Input: part model. Units: mm. Frame: model coordinates. Face numbers are marked on the shaded views. A direction names the side the tool comes from. Give positions to 0.01 mm unless a question says otherwise; leave off trailing zeros. Write each loop counter-clockwise with the first axis right and the second up, starting at its lowest first coordinate (ties: lowest second). Pieces come first, ordered by that corner, then holes. Notation, with made-up numbers: (3, 55.5) - (55, 55.5) arc R15 ccw to (55, 81.5) - close; hole circle Ø6 at (-15, 66.25). An arc over 180 degrees is marked (long way). Answer as CSV lines item,"result".
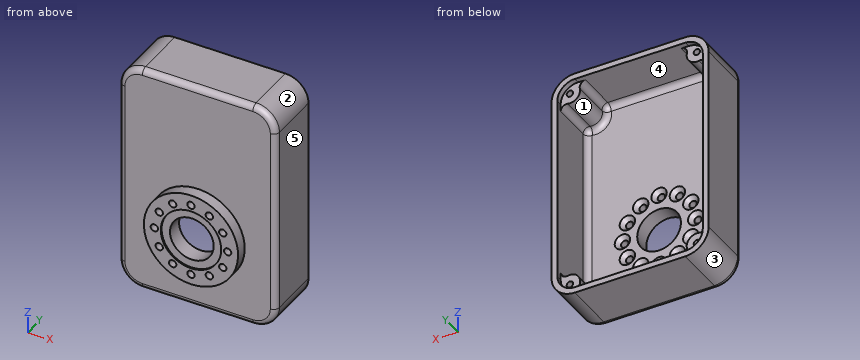
```python
from build123d import *

# Parameters (mm, degrees)
BOSS_EXTRUDE1_START           = 2.54
SKETCH4_R                     = 9.5504
BOSS_EXTRUDE1_DEPTH           = 2.54
CSK_FOR_M3_SFHCS1_D           = 3.2
CSK_FOR_M3_SFHCS1_CSINK_D     = 6.72
CSK_FOR_M3_SFHCS1_CSINK_ANGLE = 90
BOSS_EXTRUDE4_START           = 22.225
BOSS_EXTRUDE4_DEPTH           = 22.225
FILLET1_R                     = 2.54
SKETCH8_R                     = 4.445
SKETCH8_R_2                   = 1.3890625
BOSS_EXTRUDE5_DEPTH           = 19.685
FILLET3_R                     = 2.54
FILLET4_R                     = 2.54


with BuildPart() as part:
    # Sketch1 → Revolve1 (revolve)
    with BuildSketch(Plane.XY, mode=Mode.PRIVATE) as revolve1_sk:
        Polygon((-9.5504, 0), (-20.574, 0), (-20.574, -5.08), (-13.208, -5.08), (-13.208, -4.445), (-9.5504, -4.445), align=None)
    revolve(revolve1_sk.sketch.rotate(Axis((0, 0, 0), (0, 1, 0)), 270), axis=Axis((0, 0, 0), (0, 1, 0)))

    # Sketch4 → Boss-Extrude1 (add)
    with BuildSketch(Plane(origin=(0, 0, 0), x_dir=(1, 0, 0), z_dir=(0, 1, 0)).offset(BOSS_EXTRUDE1_START)):
        with BuildLine():
            Line((-24.13, -67.31), (24.13, -67.31))
            ThreePointArc((24.13, -67.31), (31.314204897, -64.334204897), (34.29, -57.15))
            Line((34.29, -57.15), (34.29, 24.13))
            ThreePointArc((34.29, 24.13), (31.314204897, 31.314204897), (24.13, 34.29))
            Line((24.13, 34.29), (-24.13, 34.29))
            ThreePointArc((-24.13, 34.29), (-31.314204897, 31.314204897), (-34.29, 24.13))
            Line((-34.29, 24.13), (-34.29, -57.15))
            ThreePointArc((-34.29, -57.15), (-31.314204897, -64.334204897), (-24.13, -67.31))
        make_face()
        Circle(SKETCH4_R, mode=Mode.SUBTRACT)
    extrude(amount=-BOSS_EXTRUDE1_DEPTH)

    # CSK for M3 SFHCS1 (through all)
    with Locations(Plane(origin=(0, 2.54, 0), x_dir=(1, 0, 0), z_dir=(0, 1, 0))):
        with Locations((-13.858138511, -8.001), (-16.002, 0), (-13.858138511, 8.001), (-8.001, 13.858138511), (0, 16.002), (8.001, 13.858138511), (13.858138511, 8.001), (16.002, 0), (13.858138511, -8.001), (8.001, -13.858138511), (0, -16.002), (-8.001, -13.858138511)):
            CounterSinkHole(CSK_FOR_M3_SFHCS1_D / 2, CSK_FOR_M3_SFHCS1_CSINK_D / 2, counter_sink_angle=CSK_FOR_M3_SFHCS1_CSINK_ANGLE)

    # Sketch6 → Boss-Extrude4 (add)
    with BuildSketch(Plane(origin=(0, 2.54, 0), x_dir=(1, 0, 0), z_dir=(0, 1, 0)).offset(BOSS_EXTRUDE4_START)):
        with BuildLine():
            Line((24.13, 34.29), (-24.13, 34.29))
            ThreePointArc((-24.13, 34.29), (-31.314204897, 31.314204897), (-34.29, 24.13))
            Line((-34.29, 24.13), (-34.29, -57.15))
            ThreePointArc((-34.29, -57.15), (-31.314204897, -64.334204897), (-24.13, -67.31))
            Line((-24.13, -67.31), (24.13, -67.31))
            ThreePointArc((24.13, -67.31), (31.314204897, -64.334204897), (34.29, -57.15))
            Line((34.29, -57.15), (34.29, 24.13))
            ThreePointArc((34.29, 24.13), (31.314204897, 31.314204897), (24.13, 34.29))
        make_face()
        with BuildLine():
            Line((24.13, 31.75), (-24.13, 31.75))
            ThreePointArc((-24.13, 31.75), (-29.518153673, 29.518153673), (-31.75, 24.13))
            Line((-31.75, 24.13), (-31.75, -57.15))
            ThreePointArc((-31.75, -57.15), (-29.518153673, -62.538153673), (-24.13, -64.77))
            Line((-24.13, -64.77), (24.13, -64.77))
            ThreePointArc((24.13, -64.77), (29.518153673, -62.538153673), (31.75, -57.15))
            Line((31.75, -57.15), (31.75, 24.13))
            ThreePointArc((31.75, 24.13), (29.518153673, 29.518153673), (24.13, 31.75))
        make_face(mode=Mode.SUBTRACT)
    extrude(amount=-BOSS_EXTRUDE4_DEPTH)

    # Fillet1
    fillet1_edges = [part.edges().sort_by_distance(p)[0] for p in [
        (-31.314204897, 0, 64.334204897),
        (0, 0, 67.31),
        (31.314204897, 0, 64.334204897),
        (34.29, 0, 16.51),
        (31.314204897, 0, -31.314204897),
        (0, 0, -34.29),
        (-31.314204897, 0, -31.314204897),
        (-34.29, 0, 16.51),
    ]]
    fillet(fillet1_edges, radius=FILLET1_R)

    # Sketch8 → Boss-Extrude5 (add)
    # profile 1 of 4: a face of its own
    with BuildSketch(Plane(origin=(0, 2.54, 0), x_dir=(1, 0, 0), z_dir=(0, 1, 0))):
        with Locations((-27.722102448, -60.742102448)):
            Circle(SKETCH8_R)
        with Locations(Location((-27.722102448, -60.742102448, 0), (0, 0, 270))):
            Circle(SKETCH8_R_2, mode=Mode.SUBTRACT)
    # profile 2 of 4: a face of its own
    with BuildSketch(Plane(origin=(0, 2.54, 0), x_dir=(1, 0, 0), z_dir=(0, 1, 0))):
        with Locations((27.722102448, -60.742102448)):
            Circle(SKETCH8_R)
        with Locations(Location((27.722102448, -60.742102448, 0), (0, 0, 270))):
            Circle(SKETCH8_R_2, mode=Mode.SUBTRACT)
    # profile 3 of 4: a face of its own
    with BuildSketch(Plane(origin=(0, 2.54, 0), x_dir=(1, 0, 0), z_dir=(0, 1, 0))):
        with Locations((27.722102448, 27.722102448)):
            Circle(SKETCH8_R)
        with Locations(Location((27.722102448, 27.722102448, 0), (0, 0, 270))):
            Circle(SKETCH8_R_2, mode=Mode.SUBTRACT)
    # profile 4 of 4: a face of its own
    with BuildSketch(Plane(origin=(0, 2.54, 0), x_dir=(1, 0, 0), z_dir=(0, 1, 0))):
        with Locations((-27.722102448, 27.722102448)):
            Circle(SKETCH8_R)
        with Locations(Location((-27.722102448, 27.722102448, 0), (0, 0, 270))):
            Circle(SKETCH8_R_2, mode=Mode.SUBTRACT)
    extrude(amount=BOSS_EXTRUDE5_DEPTH)

    # Fillet3
    # the kernel refuses this fillet: 2.54 mm, written as the material it adds along each edge
    with BuildSketch(Plane(origin=(25.571770391, 2.54, 64.632359129), x_dir=(-0.5973974080073474, 0, -0.8019453453360166), z_dir=(0, 1, 0)), Plane(origin=(31.612359129, 2.54, -25.571770391), x_dir=(-0.8019453453360167, 0, 0.5973974080073472), z_dir=(0, 1, 0)), Plane(origin=(-25.571770391, 2.54, -31.612359129), x_dir=(0.5973974080073424, 0, 0.8019453453360202), z_dir=(0, 1, 0)), Plane(origin=(-31.612359129, 2.54, 58.591770391), x_dir=(0.8019453453360194, 0, -0.5973974080073438), z_dir=(0, 1, 0))) as fillet3_piece_1:
        with BuildLine():
            CenterArc((4.719009703, 2.313416024), FILLET3_R, 143.316272758, 102.298995101)
            Line((2.682068526, 3.83080544), (2.478374408, 3.982544382))
            ThreePointArc((2.478374408, 3.982544382), (0.547235321, 1.390186295), (-0.228725099, 0.110457363))
            Line((-0.228725099, 0.110457363), (0.104866882, -0.231341602))
            ThreePointArc((0.104866882, -0.231341602), (1.83517044, 0.142521958), (3.565473998, -0.231341602))
            Line((3.565473998, -0.231341602), (3.67034088, 0))
        make_face()
    extrude(amount=19.685)
    with BuildSketch(Plane(origin=(31.612359129, 2.54, 58.591770391), x_dir=(-0.8019453453360176, 0, -0.5973974080073462), z_dir=(0, 1, 0)), Plane(origin=(25.571770391, 2.54, -31.612359129), x_dir=(-0.5973974080073442, 0, 0.801945345336019), z_dir=(0, 1, 0)), Plane(origin=(-31.612359129, 2.54, -25.571770391), x_dir=(0.8019453453360176, 0, 0.5973974080073461), z_dir=(0, 1, 0)), Plane(origin=(-25.571770391, 2.54, 64.632359129), x_dir=(0.5973974080073453, 0, -0.8019453453360182), z_dir=(0, 1, 0))) as fillet3_piece_2:
        with BuildLine():
            CenterArc((4.719009703, -2.313416024), FILLET3_R, 114.384732141, 102.298995101)
            Line((2.682068526, -3.83080544), (2.478374408, -3.982544382))
            ThreePointArc((2.478374408, -3.982544382), (0.547235321, -1.390186295), (-0.228725099, -0.110457363))
            Line((-0.228725099, -0.110457363), (0.104866882, 0.231341602))
            ThreePointArc((0.104866882, 0.231341602), (1.83517044, -0.142521958), (3.565473998, 0.231341602))
            Line((3.565473998, 0.231341602), (3.67034088, 0))
        make_face()
    extrude(amount=19.685)

    # Fillet4
    fillet4_edges = [part.edges().sort_by_distance(p)[0] for p in [
        (0, 2.54, 64.77),
        (-24.579012806, 2.54, -24.579012806),
        (-31.75, 2.54, 16.51),
        (-24.579012806, 2.54, 57.599012806),
        (24.579012806, 2.54, 57.599012806),
        (31.75, 2.54, 16.51),
        (24.579012806, 2.54, -24.579012806),
        (0, 2.54, -31.75),
        (-22.875527809, 2.54, 63.823317877),
        (-30.803317877, 2.54, 55.895527809),
        (-22.875527809, 2.54, -30.803317877),
        (-30.803317877, 2.54, -22.875527809),
        (30.803317877, 2.54, -22.875527809),
        (22.875527809, 2.54, -30.803317877),
        (30.803317877, 2.54, 55.895527809),
        (22.875527809, 2.54, 63.823317877),
    ]]
    fillet(fillet4_edges, radius=FILLET4_R)


solid = part.part
```
Item 1: Reachability of the marked faces 1 and 2 from +Z, -Z, +X, -X, +Y, -Y: full face, straight path, thin tool, end or side. Return the list, or none.
The answers:
face 1,"+Y"
face 2,"+Z, +X, +Y, -Y"
Item 2: Cut plane B-B on y = 15.75. Return the cut outline in (x, z) (3 decimals).
The answers:
outline,"(-34.29, -24.13) arc R10.16 ccw to (-24.13, -34.29) - (24.13, -34.29) arc R10.16 ccw to (34.29, -24.13) - (34.29, 57.15) arc R10.16 ccw to (24.13, 67.31) - (-24.13, 67.31) arc R10.16 ccw to (-34.29, 57.15) - close; hole (-31.75, -20.897) arc R2.54 ccw to (-28.669, -23.379) arc R4.445 cw to (-23.379, -28.669) arc R2.54 ccw to (-20.897, -31.75) - (20.897, -31.75) arc R2.54 ccw to (23.379, -28.669) arc R4.445 cw to (28.669, -23.379) arc R2.54 ccw to (31.75, -20.897) - (31.75, 53.917) arc R2.54 ccw to (28.669, 56.399) arc R4.445 cw to (23.379, 61.689) arc R2.54 ccw to (20.897, 64.77) - (-20.897, 64.77) arc R2.54 ccw to (-23.379, 61.689) arc R4.445 cw to (-28.669, 56.399) arc R2.54 ccw to (-31.75, 53.917) - close; hole circle Ø2.778 at (-27.722, -27.722); hole circle Ø2.778 at (-27.722, 60.742); hole circle Ø2.778 at (27.722, -27.722); hole circle Ø2.778 at (27.722, 60.742)"
Item 3: Contact query for flat-ended pins moving along their axis: pin 1 (5 mm diameter, centred on x = 8, z = -13.86, fed in from -Y); pin 2 (1.9 mm diameter, centred on x = -8, z = -13.86, fed in from -Y); pin 3 (2 mm diameter, centred on x = 1.5, z = 24.5, fed in from -Y); pin 4 (3 mm diameter, centred on x = 16.5, z = 42.5, fed in from +Y). Output: stop coordinate, or through.
The answers:
pin 1,"y = -5.08"
pin 2,"through"
pin 3,"y = 0"
pin 4,"y = 2.54"
Item 4: Mould query, pull axis X, two halves, no side actions, for the marked faces 3, 4 and 5. Classes: +X half, -X half, draft (parallel to the pull), parting line (faces both ways), or undercut.
The answers:
face 3,"-X half"
face 4,"undercut"
face 5,"+X half"
Item 5: Cut plane A-A on z = 0. Count the separate pieces of the cut face and the enclosed holes in it, plus the area to 3 significant figures.
The answers:
separate pieces,"4"
enclosed holes,"0"
area,"291 mm²"
Item 6: Ray query, line 1 (X direction, y = 11, z = 42); line 2 (Z direction, x = 17.5, y = 11); line 3 (Z direction, x = -7, y = 2.25). Return the intervals inside material, ascending. Write a range as from..to.
The answers:
line 1,"-34.29..-31.75, 31.75..34.29"
line 2,"-34.29..-31.75, 64.77..67.31"
line 3,"-34.27..-16.76, -10.96..-6.5, 6.5..10.96, 16.76..67.29"
